CAD build for the part. Positions are in the model's coordinates, mm. Give positions to 0.01 mm unless a question says otherwise; leave off trailing zeros. Loops run counter-clockwise (first coordinate to the right, second up) from the corner with the lowest first, then second, coordinate; pieces in that order, holes last. Notation, with made-up numbers: (-18, 46) - (30, 46) arc R21 ccw to (30, 81) - close; hole circle Ø3 at (3, 67). An arc over 180 degrees is marked (long way). Return JSON: item names as keys, results as strings.
Solid Edge part; units mm, degrees
sketch "Sketch1" plane through (0, 0, -1) normal (0, 0, 1) x (1, 0, 0)
  line L0 (-53, -49) -> (53, -49)
  line L1 (53, -49) -> (53, 32)
  line L2 (53, 32) -> (-53, 32)
  line L3 (-53, 32) -> (-53, -49)
  circle A0 centre (0, 0) radius 12.2
  circle A1 centre (-23, -43) radius 1.7
  circle A2 centre (23, -43) radius 1.7
  circle A3 centre (-23, 18) radius 1.7
  circle A4 centre (23, 18) radius 1.7
  circle A5 centre (-45, -25) radius 1.7
  circle A6 centre (45, -25) radius 1.7
  circle A7 centre (-45, 25) radius 1.7
  circle A8 centre (45, 25) radius 1.7
extrude "ExtrudedProtrusion_1" add sketch "Sketch1" along normal blind 4
extrude "ExtrudedProtrusion_2" [suppressed]
extrude "ExtrudedProtrusion_3" [suppressed]
1. Cut at A-A, the plane x = -45. Write the cut outline in (y, z).
Values follow:
{"outline": "(-49, -1) - (-26.7, -1) - (-26.7, 3) - (-49, 3) - close; (-23.3, -1) - (23.3, -1) - (23.3, 3) - (-23.3, 3) - close; (26.7, -1) - (32, -1) - (32, 3) - (26.7, 3) - close"}
2. Cut at C-C, the plane y = 25. Write the cut outline in (x, z), plus the area to 3 significant figures.
Values follow:
{"outline": "(-53, -1) - (-46.7, -1) - (-46.7, 3) - (-53, 3) - close; (-43.3, -1) - (43.3, -1) - (43.3, 3) - (-43.3, 3) - close; (46.7, -1) - (53, -1) - (53, 3) - (46.7, 3) - close", "area": "397 mm²"}
3. Drill centre lines: probe 1 along Y at (x, z) = (-45, 0); probe 2 along Y at (x, z) = (-23, 0.9); probe 3 along Y at (x, z) = (-10, 1.45). Where is each one in solid material? Low to high.
Values follow:
{"probe 1": "y = -49 to -26.7, -23.3 to 23.3, 26.7 to 32", "probe 2": "y = -49 to -44.7, -41.3 to 16.3, 19.7 to 32", "probe 3": "y = -49 to -6.99, 6.99 to 32"}
4. Cut at D-D, the plane x = 0. Write the cut outline in (y, z), plus the area to 3 significant figures.
Values follow:
{"outline": "(-49, -1) - (-12.2, -1) - (-12.2, 3) - (-49, 3) - close; (12.2, -1) - (32, -1) - (32, 3) - (12.2, 3) - close", "area": "226 mm²"}
5. Pull direction X, two halves, no side cores. Call faces 1 (the face through (-1, -49, 1)), 2 (the face through (-46.25, -26.15, 0.97)), 3 (the face through (-53, -8, 1)), 4 (the face through (53, -9, 1)): +X half, -X half, draft (parallel to the pull), parting line (faces both ways), or undercut.
Values follow:
{"face 1": "draft", "face 2": "undercut", "face 3": "-X half", "face 4": "+X half"}
6. Cut at B-B, the plane z = 0.3. Give the number of separate pieces and of enclosed holes in the cut face, plus the area to 3 significant figures.
Values follow:
{"separate pieces": "1", "enclosed holes": "9", "area": "8,050 mm²"}
